Part model, mm, in its own coordinate system. Face numbers are marked on the shaded views. A direction names the side the tool comes from. Give positions to 0.01 mm unless a question says otherwise; leave off trailing zeros. Order: outer loops, then holes, each group sorted by start corner. A loop starts at its lowest first (then second) coordinate and runs counter-clockwise, first axis right, second up. Notation, with made-up numbers: (-37, 88) - (-1, 88) arc R22 cw to (-1, 114) - close; hole circle Ø8 at (62, -30.75). An arc over 180 degrees is marked (long way). Use one line per item in the form item = value. Start each with the question number.
1. Band-saw the part on B-B, the plane y = 1.8. List the corners of the cut face in (x, z).
2. Drill centre lines: line 1 (X direction, y = 1.85, z = 23.75); line 2 (X direction, y = 2.1, z = 1.75); line 3 (X direction, y = 3.35, z = 18.75). Where is each one in solid material? Low to high.
3. Band-saw the part on D-D, the plane z = 18.5. List the corners of the cut face in (x, y), plus the area to 3 significant figures.
4. Pull direction X, two halves, no side cores. Call the marked faces 1, 2, 3 and 4: +X half, -X half, draft (parallel to the pull), parting line (faces both ways), or undercut.
5. Band-saw the part on A-A, the plane z = 23.75. List the corners of the cut face in (x, y).
6. Tool access for the marked faces 5, 6, 7 and 8: list every direction of +Z, -Z, +X, -X, +Y, -Y with a clear straight run to the whole face (end or side of a thin tool).
7. Band-saw the part on C-C, the plane x = 33. List the corners of the cut face in (y, z), plus the area to 3 significant figures.
8. Pin check, flat tips, straight feed: P1, Ø2, axis at x = -2, y = 1, coming from the -Z side; P2, Ø1.2, axis at y = 3, z = 21, coming from the +X side; P3, Ø1, axis at x = 20.5, z = 10, coming from the -Y side; P4, Ø1.2, axis at y = 1.5, z = 21, coming from the -X side. Stop position of each tip, or through.
from build123d import *

# Parameters (mm, degrees)
SKETCH1_W           = 32.5
SKETCH1_H           = 25
BOSS_EXTRUDE1_DEPTH = 4
SKETCH2_R           = 2.25
SKETCH2_W           = 4.5
SKETCH2_H           = 2.25
CUT_EXTRUDE5_DEPTH  = 5
SKETCH3_W           = 4
SKETCH3_H           = 10
BOSS_EXTRUDE2_DEPTH = 4
SKETCH4_W           = 10
SKETCH4_H           = 4
CUT_EXTRUDE6_DEPTH  = 5


with BuildPart() as part:
    # Sketch1 → Boss-Extrude1 (new body)
    with BuildSketch(Plane(origin=(0, 0, 0), x_dir=(1, 0, 0), z_dir=(0, 1, 0))):
        with Locations((16.25, -12.5)):
            Rectangle(SKETCH1_W, SKETCH1_H)
    extrude(amount=BOSS_EXTRUDE1_DEPTH)

    # Sketch2 → Cut-Extrude5 (cut, through all)
    with BuildSketch(Plane(origin=(0, 4, 0), x_dir=(1, 0, 0), z_dir=(0, 1, 0))):
        with Locations((16.25, -2.25)):
            Circle(SKETCH2_R)
        with Locations((16.25, -1.125)):
            Rectangle(SKETCH2_W, SKETCH2_H)
    extrude(amount=-CUT_EXTRUDE5_DEPTH, mode=Mode.SUBTRACT)

    # Sketch3 → Boss-Extrude2 (add, through all)
    with BuildSketch(Plane(origin=(0, 4, 0), x_dir=(1, 0, 0), z_dir=(0, 1, 0))):
        with Locations((-2, -12.5)):
            Rectangle(SKETCH3_W, SKETCH3_H)
        with Locations((34.5, -12.5)):
            Rectangle(SKETCH3_W, SKETCH3_H)
    extrude(amount=-BOSS_EXTRUDE2_DEPTH)

    # Sketch4 → Cut-Extrude6 (cut, through all)
    with BuildSketch(Plane(origin=(0, 4, 0), x_dir=(1, 0, 0), z_dir=(0, 1, 0))):
        with Locations((16.25, -23)):
            Rectangle(SKETCH4_W, SKETCH4_H)
    extrude(amount=-CUT_EXTRUDE6_DEPTH, mode=Mode.SUBTRACT)


solid = part.part
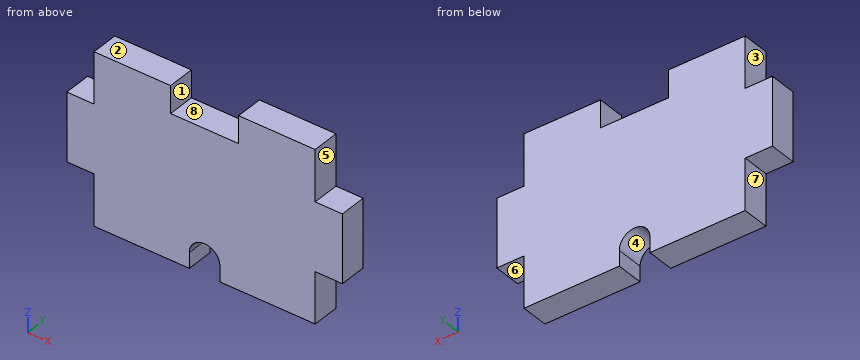
From the geometry:
q1.outline = (-4, 7.5) - (0, 7.5) - (0, 0) - (14, 0) - (14, 2.25) arc R2.25 cw to (18.5, 2.25) - (18.5, 0) - (32.5, 0) - (32.5, 7.5) - (36.5, 7.5) - (36.5, 17.5) - (32.5, 17.5) - (32.5, 25) - (21.25, 25) - (21.25, 21) - (11.25, 21) - (11.25, 25) - (0, 25) - (0, 17.5) - (-4, 17.5) - close
q2.line_1 = 0 to 11.25, 21.25 to 32.5
q2.line_2 = 0 to 14, 18.5 to 32.5
q2.line_3 = 0 to 32.5
q3.outline = (0, 0) - (32.5, 0) - (32.5, 4) - (0, 4) - close
q3.area = 130 mm²
q4.face_1 = undercut
q4.face_2 = draft
q4.face_3 = -X half
q4.face_4 = undercut
q5.outline = (0, 0) - (11.25, 0) - (11.25, 4) - (0, 4) - close; (21.25, 0) - (32.5, 0) - (32.5, 4) - (21.25, 4) - close
q6.face_5 = +Z, +X, +Y, -Y
q6.face_6 = -Z, +X, +Y, -Y
q6.face_7 = -Z, -X, +Y, -Y
q6.face_8 = +Z, +Y, -Y
q7.outline = (0, 7.5) - (4, 7.5) - (4, 17.5) - (0, 17.5) - close
q7.area = 40.0 mm²
q8.P1 = 7.5
q8.P2 = 32.5
q8.P3 = 0
q8.P4 = 0
